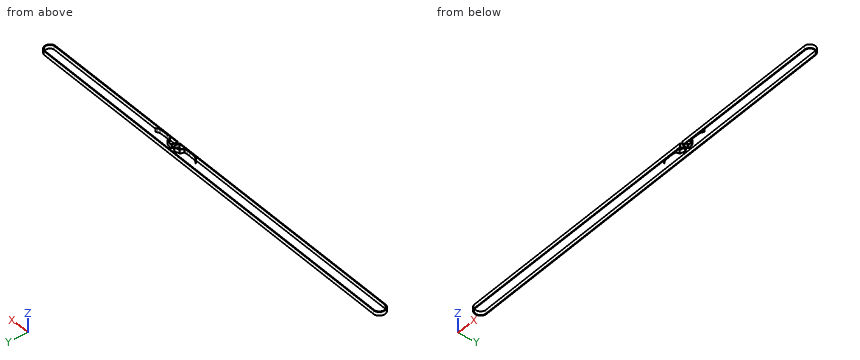
Autodesk Inventor part; units mm, degrees
ref_plane "YZ Plane" through (0, 0, 0) normal (1, 0, 0) x (0, 1, 0)
ref_plane "XZ Plane" through (0, 0, 0) normal (0, 1, 0) x (-1, 0, 0)
ref_plane "XY Plane" through (0, 0, 0) normal (0, 0, 1) x (1, 0, 0)
ref_plane "Work Plane1" through (0, 0, 0) normal (0, 0, 1) x (1, 0, 0)
sketch "Sketch1" plane through (0, 0, 0) normal (0, 0, 1) x (1, 0, 0)
  arc A0 (24.6543, 36.9901) -> (24.6581, 49.8888) centre (24.6562, 43.4394) ccw
  arc A1 (-523.0049, 50.5993) -> (-523.009, 36.5993) centre (-523.014, 43.5993) ccw
  line L0 (-523.009, 36.5993) -> (24.8958, 36.9945)
  line L1 (24.9813, 49.8806) -> (-523.0049, 50.5993)
  line L2 (-523.0083, 35.5993) -> (24.9141, 35.9946)
  arc A2 (24.655, 35.9901) -> (24.666, 50.8888) centre (24.6562, 43.4394) ccw
  arc A3 (-523.0035, 51.5993) -> (-523.0083, 35.5993) centre (-523.014, 43.5993) ccw
  line L3 (-523.0035, 51.5993) -> (25.0062, 50.8806)
  point P0 (0, 0)
  dimension "d0" = 1
ref_plane "Work Plane2" through (0, 0, 6) normal (0, 0, 1) x (1, 0, 0)
sketch "Sketch2" plane through (0, 0, 6) normal (0, 0, 1) x (1, 0, 0)
  line L0 (-523.0049, 50.5993) -> (24.9813, 49.8806)
  arc A0 (26.1347, 37.1513) -> (24.9813, 49.8806) centre (24.6937, 43.4377) ccw
  arc A1 (-523.0049, 50.5993) -> (-523.0019, 36.5993) centre (-523.0069, 43.5993) ccw
  line L1 (-523.0501, 35.5895) -> (-182.2036, 35.8354)
  arc A2 (24.8737, 35.9804) -> (24.9644, 50.8708) centre (24.674, 43.4271) ccw
  line L2 (24.9644, 50.8708) -> (-523.0453, 51.5895)
  arc A3 (-523.0453, 51.5895) -> (-523.0501, 35.5895) centre (-523.0477, 43.5895) ccw
  line L3 (26.1347, 37.1513) -> (-177.3524, 36.8243)
  line L4 (26.1347, 37.1513) -> (-177.3524, 36.8243)
  line L5 (-177.55, 35.8233) -> (24.8737, 35.9804)
  line L6 (-182.3943, 36.845) -> (-523.0019, 36.5993)
  line L7 (-182.3943, 36.845) -> (-523.0019, 36.5993)
  line L8 (-182.3943, 36.845) -> (-523.009, 36.5993)
  arc A4 (-175.5981, 44.0056) -> (-177.8793, 42.0255) centre (-175.8793, 42.0255) ccw
  line L9 (-177.8793, 42.0255) -> (-177.8793, 38.1674)
  line L10 (-168.9783, 38.1674) -> (-177.8793, 38.1674)
  arc A5 (-168.9783, 38.1674) -> (-168.8741, 38.8755) centre (-169.5783, 38.6174) ccw
  line L11 (-168.8741, 38.8755) -> (-169.5014, 41.4937)
  arc A6 (-169.5014, 41.4937) -> (-170.852, 42.9373) centre (-171.4464, 41.0276) ccw
  arc A7 (-170.852, 42.9373) -> (-175.5981, 44.0056) centre (-179.8602, 13.9956) ccw
  arc A8 (-181.8793, 42.02) -> (-184.1633, 43.9998) centre (-183.8793, 42.02) ccw
  arc A9 (-184.1633, 43.9998) -> (-188.8754, 42.9351) centre (-179.8602, 13.9956) ccw
  arc A10 (-188.8754, 42.9351) -> (-190.223, 41.5019) centre (-188.2805, 41.0256) ccw
  line L12 (-190.223, 41.5019) -> (-190.8453, 38.9643)
  arc A11 (-190.8453, 38.9643) -> (-190.7804, 38.1674) centre (-190.1804, 38.6174) ccw
  line L13 (-181.8793, 38.1674) -> (-190.7804, 38.1674)
  line L14 (-181.8793, 42.02) -> (-181.8793, 38.1674)
  line L15 (-177.3524, 36.8243) -> (-177.8746, 37.7286)
  line L16 (-177.8746, 37.7286) -> (-178.2063, 38.5555)
  line L17 (-178.2063, 38.5555) -> (-178.2078, 40.6305)
  line L18 (-178.2078, 40.6305) -> (-178.209, 42.3362)
  line L19 (-178.209, 42.3362) -> (-177.737, 43.3845)
  line L20 (-177.737, 43.3845) -> (-177.1904, 43.8398)
  line L21 (-177.1904, 43.8398) -> (-176.2125, 44.2321)
  line L22 (-176.2125, 44.2321) -> (-175.2227, 44.2328)
  line L23 (-175.2227, 44.2328) -> (-170.4599, 42.9351)
  line L24 (-170.4599, 42.9351) -> (-169.9859, 42.5772)
  line L25 (-169.9859, 42.5772) -> (-169.4819, 41.9721)
  line L26 (-169.4819, 41.9721) -> (-168.629, 38.4129)
  line L27 (-168.629, 38.4129) -> (-167.76, 37.7567)
  line L28 (-167.76, 37.7567) -> (-165.9159, 37.2737)
  line L29 (-165.9159, 37.2737) -> (-163.1275, 36.9945)
  line L30 (-163.1275, 36.9945) -> (-160.3695, 36.9965)
  line L31 (-160.3695, 36.9965) -> (-151.627, 37.2737)
  line L32 (-151.627, 37.2737) -> (-150.5918, 37.5217)
  line L33 (-150.5918, 37.5217) -> (-148.0211, 38.5527)
  line L34 (-148.0211, 38.5527) -> (-146.3842, 39.9163)
  line L35 (-146.3842, 39.9163) -> (-146.6143, 40.1925)
  line L36 (-146.6143, 40.1925) -> (-148.2512, 38.8289)
  line L37 (-148.2512, 38.8289) -> (-150.6724, 37.8579)
  line L38 (-150.6724, 37.8579) -> (-151.8853, 37.5672)
  line L39 (-151.8853, 37.5672) -> (-160.472, 37.295)
  line L40 (-160.472, 37.295) -> (-163.1702, 37.4311)
  line L41 (-163.1702, 37.4311) -> (-165.8102, 37.5643)
  line L42 (-165.8102, 37.5643) -> (-167.6157, 38.0372)
  line L43 (-167.6157, 38.0372) -> (-168.2752, 38.8289)
  line L44 (-168.2752, 38.8289) -> (-169.2827, 42.138)
  line L45 (-169.2827, 42.138) -> (-169.6866, 42.8265)
  line L46 (-169.6866, 42.8265) -> (-170.4021, 43.1486)
  line L47 (-170.4021, 43.1486) -> (-175.2236, 44.4623)
  line L48 (-175.2236, 44.4623) -> (-175.9859, 44.5387)
  line L49 (-175.9859, 44.5387) -> (-176.8242, 44.3378)
  line L50 (-176.8242, 44.3378) -> (-177.6272, 43.8055)
  line L51 (-177.6272, 43.8055) -> (-178.135, 43.3825)
  line L52 (-178.135, 43.3825) -> (-178.4245, 42.5752)
  line L53 (-178.4245, 42.5752) -> (-178.6341, 40.4815)
  line L54 (-178.6341, 40.4815) -> (-178.4776, 38.0352)
  line L55 (-178.4776, 38.0352) -> (-177.55, 35.8233)
  line L56 (-177.8793, 40.4835) -> (-181.8793, 40.4835)
  line L57 (-179.8793, 40.4835) -> (-179.8793, 39.2603)
  arc A12 (-181.8793, 42.0255) -> (-184.1606, 44.0056) centre (-183.8793, 42.0255) ccw
  line L58 (-181.8793, 42.0255) -> (-181.8793, 38.1674)
  line L59 (-190.7804, 38.1674) -> (-181.8793, 38.1674)
  arc A13 (-190.8846, 38.8755) -> (-190.7804, 38.1674) centre (-190.1804, 38.6174) ccw
  line L60 (-190.8846, 38.8755) -> (-190.2572, 41.4937)
  arc A14 (-188.9067, 42.9373) -> (-190.2572, 41.4937) centre (-188.3123, 41.0276) ccw
  arc A15 (-184.1606, 44.0056) -> (-188.9067, 42.9373) centre (-179.8985, 13.9956) ccw
  line L61 (-182.3943, 36.845) -> (-181.8841, 37.7286)
  line L62 (-181.8841, 37.7286) -> (-181.5524, 38.5555)
  line L63 (-181.5524, 38.5555) -> (-181.5509, 40.6305)
  line L64 (-181.5509, 40.6305) -> (-181.5497, 42.3362)
  line L65 (-181.5497, 42.3362) -> (-182.0217, 43.3845)
  line L66 (-182.0217, 43.3845) -> (-182.5683, 43.8398)
  line L67 (-182.5683, 43.8398) -> (-183.5462, 44.2321)
  line L68 (-183.5462, 44.2321) -> (-184.536, 44.2328)
  line L69 (-184.536, 44.2328) -> (-189.2987, 42.9351)
  line L70 (-189.2987, 42.9351) -> (-189.7728, 42.5772)
  line L71 (-189.7728, 42.5772) -> (-190.2768, 41.9721)
  line L72 (-190.2768, 41.9721) -> (-191.1297, 38.4129)
  line L73 (-191.1297, 38.4129) -> (-191.9987, 37.7567)
  line L74 (-191.9987, 37.7567) -> (-193.8428, 37.2737)
  line L75 (-193.8428, 37.2737) -> (-196.6311, 36.9945)
  line L76 (-196.6311, 36.9945) -> (-199.3891, 36.9965)
  line L77 (-199.3891, 36.9965) -> (-208.1317, 37.2737)
  line L78 (-208.1317, 37.2737) -> (-209.1668, 37.5217)
  line L79 (-209.1668, 37.5217) -> (-211.7376, 38.5527)
  line L80 (-211.7376, 38.5527) -> (-213.3745, 39.9163)
  line L81 (-213.3745, 39.9163) -> (-213.1444, 40.1925)
  line L82 (-213.1444, 40.1925) -> (-211.5075, 38.8289)
  line L83 (-211.5075, 38.8289) -> (-209.0863, 37.8579)
  line L84 (-209.0863, 37.8579) -> (-207.8734, 37.5672)
  line L85 (-207.8734, 37.5672) -> (-199.2867, 37.295)
  line L86 (-199.2867, 37.295) -> (-196.5885, 37.4311)
  line L87 (-196.5885, 37.4311) -> (-193.9485, 37.5643)
  line L88 (-193.9485, 37.5643) -> (-192.143, 38.0372)
  line L89 (-192.143, 38.0372) -> (-191.4835, 38.8289)
  line L90 (-191.4835, 38.8289) -> (-190.476, 42.138)
  line L91 (-190.476, 42.138) -> (-190.0721, 42.8265)
  line L92 (-190.0721, 42.8265) -> (-189.3566, 43.1486)
  line L93 (-189.3566, 43.1486) -> (-184.5351, 44.4623)
  line L94 (-184.5351, 44.4623) -> (-183.7728, 44.5387)
  line L95 (-183.7728, 44.5387) -> (-182.9345, 44.3378)
  line L96 (-182.9345, 44.3378) -> (-182.1314, 43.8055)
  line L97 (-182.1314, 43.8055) -> (-181.6237, 43.3825)
  line L98 (-181.6237, 43.3825) -> (-181.3342, 42.5752)
  line L99 (-181.3342, 42.5752) -> (-181.1246, 40.4815)
  line L100 (-181.1246, 40.4815) -> (-181.2811, 38.0352)
  line L101 (-181.2811, 38.0352) -> (-182.2036, 35.8354)
  point P0 (-182.2087, 35.8233)
  point P1 (-182.4063, 36.8243)
extrude "Extrusion2" add sketch "Sketch2" against normal blind 5 contours A1 L6 L61 L62 L63 L56 L100 L101 L1 A3 L2 A2 L5 L55 L54 L17 L16 L15 L3 A0 L0 | L56 L53 L52 L51 L50 L49 L48 L47 L46 L45 L44 L43 L42 L41 L40 L39 L38 L37 L36 L35 L34 L33 L32 L31 L30 L29 L28 L27 L26 L25 L24 L23 L22 L21 L20 L19 L18 L17 | L63 L64 L65 L66 L67 L68 L69 L70 L71 L72 L73 L74 L75 L76 L77 L78 L79 L80 L81 L82 L83 L84 L85 L86 L87 L88 L89 L90 L91 L92 L93 L94 L95 L96 L97 L98 L99 L56
properties part number "XBELT"
Read the model definition and answer for the solid it produces. Units are mm, in the model's axes. Coordinates: 2 decimals unless noted, no trailing zeros. Loops run counter-clockwise (first coordinate to the right, second up) from the corner with the lowest first, then second, coordinate; pieces in that order, holes last.
(1) Flat-ended cylindrical pins translate along their axes: pin 1 Ø6 at (x, y) = (-117, 41) entering from +Z; pin 2 Ø1 at (y, z) = (47, 4) entering from +X; pin 3 Ø1 at (y, z) = (41, 3) entering from +X; pin 4 Ø2 at (x, z) = (-356, 5.5) entering from -Y. Find the tip coordinate at first contact, or state that the pin passes through.
Solution:
pin 1: passes through
pin 2: stops at x = 31.46
pin 3: stops at x = 31.87
pin 4: stops at y = 35.71
(2) The part is cut by section A-A (x = -244). Determine the outline of the cut face in (y, z), and give its area (4 significant figures).
Solution:
outline: (35.79, 1) - (36.8, 1) - (36.8, 6) - (35.79, 6) - close; (50.23, 1) - (51.22, 1) - (51.22, 6) - (50.23, 6) - close
area: 10.00 mm2
(3) The part is cut by section B-B (y = 47). Determine the outline of the cut face in (x, z), and give its area (3 significant figures).
Solution:
outline: (-530.28, 1) - (-529.13, 1) - (-529.13, 6) - (-530.28, 6) - close; (30.07, 1) - (31.21, 1) - (31.21, 6) - (30.07, 6) - close
area: 11.5 mm2
(4) Consider line 1 along X through (y, z) = (42.75, 2.15); line 2 along Y through (x, z) = (-164.5, 5.4); line 3 along Y through (x, z) = (-212, 4.75). Determine where each line is inside the solid, lowest interval first.
Solution:
line 1: x = -531 to -529.96, -190.12 to -189.54, -181.74 to -181.4, -178.36 to -178.02, -170.21 to -169.64, 31.11 to 32.09
line 2: y = 35.83 to 36.84, 37.13 to 37.5, 50.13 to 51.12
line 3: y = 35.81 to 36.82, 38.77 to 39.24, 50.19 to 51.18
